Input: part model. Units: mm. Frame: model coordinates. Coordinates: 2 decimals unless noted, no trailing zeros. Loops run counter-clockwise (first coordinate to the right, second up) from the corner with the lowest first, then second, coordinate; pieces in that order, holes last. Notation, with made-up numbers: (71, -14) - (124, -14) arc R29 ccw to (124, 19) - close; hole circle Ø3 at (-32.5, 61). An arc over 180 degrees is marked (long way). Use one line per item in the form item = value.
from build123d import *

# Parameters (mm, degrees)
SKETCH_1_W          = 20
SKETCH_1_H          = 21
EXTRUDE_1_DEPTH     = 42
CUT_EXTRUDE_1_REACH = 53.039
SKETCH_2_R          = 2.15
FILLET_1_R          = 2


with BuildPart() as part:
    # 草图1 → 凸台-拉伸1 (new body)
    with BuildSketch(Plane.XY):
        with Locations((-10, 10.5)):
            Rectangle(SKETCH_1_W, SKETCH_1_H)
    extrude(amount=EXTRUDE_1_DEPTH)

    # 草图2 → 切除-拉伸1 (cut, up to next)
    with BuildSketch(Plane(origin=(0, 21, 0), x_dir=(1, 0, 0), z_dir=(0, 1, 0)), mode=Mode.PRIVATE) as cut_extrude_1_sk1:
        with Locations(Location((-10, -5, 0), (0, 0, 180))):
            Circle(SKETCH_2_R)
    cut_extrude_1_tool1 = extrude(cut_extrude_1_sk1.sketch, amount=-CUT_EXTRUDE_1_REACH, mode=Mode.PRIVATE) & part.part
    # 草图2 → 切除-拉伸1 (cut, up to next)
    with BuildSketch(Plane(origin=(0, 21, 0), x_dir=(1, 0, 0), z_dir=(0, 1, 0)), mode=Mode.PRIVATE) as cut_extrude_1_sk2:
        with Locations(Location((-10, -37, 0), (0, 0, 180))):
            Circle(SKETCH_2_R)
    cut_extrude_1_tool2 = extrude(cut_extrude_1_sk2.sketch, amount=-CUT_EXTRUDE_1_REACH, mode=Mode.PRIVATE) & part.part
    add(cut_extrude_1_tool1.solids().sort_by_distance((-10, 21, 5))[0], mode=Mode.SUBTRACT)
    add(cut_extrude_1_tool2.solids().sort_by_distance((-10, 21, 37))[0], mode=Mode.SUBTRACT)

    # 圆角1
    fillet_1_edges = [part.edges().sort_by_distance(p)[0] for p in [
        (-20, 10.5, 42),
        (0, 10.5, 42),
        (-20, 10.5, 0),
        (0, 10.5, 0),
        (-20, 21, 21),
        (0, 21, 21),
    ]]
    fillet(fillet_1_edges, radius=FILLET_1_R)


solid = part.part
Q1. Ray query, line 1 along Z through (x, y) = (-10, 10.75); line 2 along Z through (x, y) = (-11, 4.5); line 3 along X through (y, z) = (13, 37.5). Return the intervals inside material, ascending. Write a range as [from, to].
Check values:
line_1 = [0, 2.85], [7.15, 34.85], [39.15, 42]
line_2 = [0, 3.1], [6.9, 35.1], [38.9, 42]
line_3 = [-20, -12.09], [-7.91, 0]
Q2. Cut plane B-B, the plane z = 37. Return loops of the section in (x, y), then the cut area to 3 significant figures.
Check values:
outline = (-20, 0) - (-12.15, 0) - (-12.15, 21) - (-18, 21) arc R2 ccw to (-20, 19) - close; (-7.85, 0) - (0, 0) - (0, 19) arc R2 ccw to (-2, 21) - (-7.85, 21) - close
area = 328 mm²
Q3. Cut plane A-A, the plane x = -10. Return loops of the section in (y, z), then the cut area to 3 significant figures.
Check values:
outline = (0, 0) - (21, 0) - (21, 2.85) - (0, 2.85) - close; (0, 7.15) - (21, 7.15) - (21, 34.85) - (0, 34.85) - close; (0, 39.15) - (21, 39.15) - (21, 42) - (0, 42) - close
area = 701 mm²
Q4. Pull-direction query (X, two-part tool) for faces 1 (the flat face through (-10, 11, 42)), 2 (the cylindrical face through (-19.43, 10.65, 41.4)), 3 (the cylindrical face through (-9.72, 10.65, 7.13)), 4 (the cylindrical face through (-9.72, 10.65, 39.13)); classes: pulls with the +X half, pulls with the -X half, needs draft (parallel to the pull), parting line crosses it, or undercut.
Check values:
face_1 = needs draft
face_2 = pulls with the -X half
face_3 = undercut
face_4 = undercut
Q5. Cut plane D-D, the plane z = 4.5. Return loops of the section in (x, y).
Check values:
outline = (-20, 0) - (-12.09, 0) - (-12.09, 21) - (-18, 21) arc R2 ccw to (-20, 19) - close; (-7.91, 0) - (0, 0) - (0, 19) arc R2 ccw to (-2, 21) - (-7.91, 21) - close
Q6. Cut plane C-C, the plane y = 11.75. Return loops of the section in (x, z), then the cut area to 3 significant figures.
Check values:
outline = (-20, 2) arc R2 ccw to (-18, 0) - (-2, 0) arc R2 ccw to (0, 2) - (0, 40) arc R2 ccw to (-2, 42) - (-18, 42) arc R2 ccw to (-20, 40) - close; hole circle Ø4.3 at (-10, 5); hole circle Ø4.3 at (-10, 37)
area = 808 mm²
